The listing builds one solid part. Answer for the finished solid, in the listing's coordinates (mm). Coordinates: 2 decimals unless noted, no trailing zeros. Loops run counter-clockwise (first coordinate to the right, second up) from the corner with the lowest first, then second, coordinate; pieces in that order, holes last. Notation, with made-up numbers: (61, 11) - (74, 11) arc R6 cw to (74, 18) - close; hole circle Ø9 at (78, -38). An arc over 180 degrees is marked (long way). Use one line per item in the form item = value. Start each with the question number.
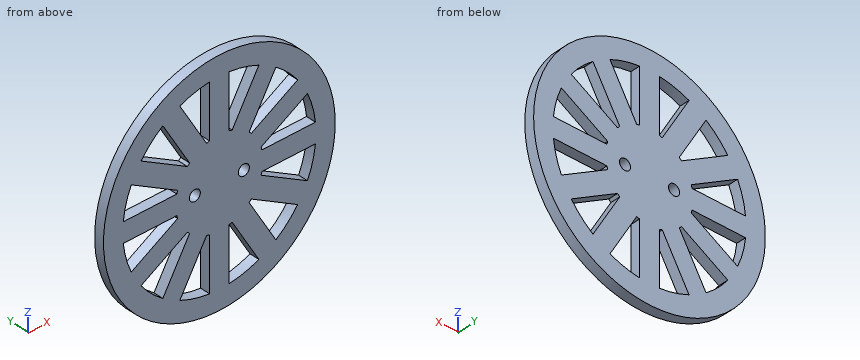
```python
from build123d import *

# Parameters (mm, degrees)
SKETCH1_R           = 30
SKETCH1_R_2         = 1.4224
BOSS_EXTRUDE1_DEPTH = 2.54


with BuildPart() as part:
    # Sketch1 → Boss-Extrude1 (new body)
    with BuildSketch(Plane(origin=(0, 0, 0), x_dir=(1, 0, 0), z_dir=(0, 1, 0))):
        Circle(SKETCH1_R)
        with BuildLine():
            ThreePointArc((3.308860999, 10.811115366), (2.926244071, 10.920891548), (2.54, 11.01713105))
            Line((2.54, 11.01713105), (2.54, 24.870633323))
            ThreePointArc((2.54, 24.870633323), (6.470476137, 24.148145694), (10.235612136, 22.808600266))
            Line((10.235612136, 22.808600266), (3.308860999, 10.811115366))
        make_face(mode=Mode.SUBTRACT)
        with BuildLine():
            ThreePointArc((8.271115366, 7.708270051), (7.994647477, 7.994647477), (7.708270051, 8.271115366))
            Line((7.708270051, 8.271115366), (14.635021187, 20.268600266))
            ThreePointArc((14.635021187, 20.268600266), (17.677669557, 17.677669557), (20.268600266, 14.635021187))
            Line((20.268600266, 14.635021187), (8.271115366, 7.708270051))
        make_face(mode=Mode.SUBTRACT)
        with BuildLine():
            ThreePointArc((11.01713105, 2.54), (10.920891548, 2.926244071), (10.811115366, 3.308860999))
            Line((10.811115366, 3.308860999), (22.808600266, 10.235612136))
            ThreePointArc((22.808600266, 10.235612136), (24.148145694, 6.470476137), (24.870633323, 2.54))
            Line((24.870633323, 2.54), (11.01713105, 2.54))
        make_face(mode=Mode.SUBTRACT)
        with BuildLine():
            ThreePointArc((10.811115366, -3.308860999), (10.920891548, -2.926244071), (11.01713105, -2.54))
            Line((11.01713105, -2.54), (24.870633323, -2.54))
            ThreePointArc((24.870633323, -2.54), (24.148145694, -6.470476137), (22.808600266, -10.235612136))
            Line((22.808600266, -10.235612136), (10.811115366, -3.308860999))
        make_face(mode=Mode.SUBTRACT)
        with BuildLine():
            ThreePointArc((7.708270051, -8.271115366), (7.994647477, -7.994647477), (8.271115366, -7.708270051))
            Line((8.271115366, -7.708270051), (20.268600266, -14.635021187))
            ThreePointArc((20.268600266, -14.635021187), (17.677669557, -17.677669557), (14.635021187, -20.268600266))
            Line((14.635021187, -20.268600266), (7.708270051, -8.271115366))
        make_face(mode=Mode.SUBTRACT)
        with BuildLine():
            ThreePointArc((2.54, -11.01713105), (2.926244071, -10.920891548), (3.308860999, -10.811115366))
            Line((3.308860999, -10.811115366), (10.235612136, -22.808600266))
            ThreePointArc((10.235612136, -22.808600266), (6.470476137, -24.148145694), (2.54, -24.870633323))
            Line((2.54, -24.870633323), (2.54, -11.01713105))
        make_face(mode=Mode.SUBTRACT)
        with BuildLine():
            ThreePointArc((-3.308860999, -10.811115366), (-2.926244071, -10.920891548), (-2.54, -11.01713105))
            Line((-2.54, -11.01713105), (-2.54, -24.870633323))
            ThreePointArc((-2.54, -24.870633323), (-6.470476137, -24.148145694), (-10.235612136, -22.808600266))
            Line((-10.235612136, -22.808600266), (-3.308860999, -10.811115366))
        make_face(mode=Mode.SUBTRACT)
        with BuildLine():
            ThreePointArc((-8.271115366, -7.708270051), (-7.994647477, -7.994647477), (-7.708270051, -8.271115366))
            Line((-7.708270051, -8.271115366), (-14.635021187, -20.268600266))
            ThreePointArc((-14.635021187, -20.268600266), (-17.677669557, -17.677669557), (-20.268600266, -14.635021187))
            Line((-20.268600266, -14.635021187), (-8.271115366, -7.708270051))
        make_face(mode=Mode.SUBTRACT)
        with BuildLine():
            ThreePointArc((-11.01713105, -2.54), (-10.920891548, -2.926244071), (-10.811115366, -3.308860999))
            Line((-10.811115366, -3.308860999), (-22.808600266, -10.235612136))
            ThreePointArc((-22.808600266, -10.235612136), (-24.148145694, -6.470476137), (-24.870633323, -2.54))
            Line((-24.870633323, -2.54), (-11.01713105, -2.54))
        make_face(mode=Mode.SUBTRACT)
        with BuildLine():
            ThreePointArc((-10.811115366, 3.308860999), (-10.920891548, 2.926244071), (-11.01713105, 2.54))
            Line((-11.01713105, 2.54), (-24.870633323, 2.54))
            ThreePointArc((-24.870633323, 2.54), (-24.148145694, 6.470476137), (-22.808600266, 10.235612136))
            Line((-22.808600266, 10.235612136), (-10.811115366, 3.308860999))
        make_face(mode=Mode.SUBTRACT)
        with BuildLine():
            ThreePointArc((-7.708270051, 8.271115366), (-7.994647477, 7.994647477), (-8.271115366, 7.708270051))
            Line((-8.271115366, 7.708270051), (-20.268600266, 14.635021187))
            ThreePointArc((-20.268600266, 14.635021187), (-17.677669557, 17.677669557), (-14.635021187, 20.268600266))
            Line((-14.635021187, 20.268600266), (-7.708270051, 8.271115366))
        make_face(mode=Mode.SUBTRACT)
        with BuildLine():
            ThreePointArc((-2.54, 11.01713105), (-2.926244071, 10.920891548), (-3.308860999, 10.811115366))
            Line((-3.308860999, 10.811115366), (-10.235612136, 22.808600266))
            ThreePointArc((-10.235612136, 22.808600266), (-6.470476137, 24.148145694), (-2.54, 24.870633323))
            Line((-2.54, 24.870633323), (-2.54, 11.01713105))
        make_face(mode=Mode.SUBTRACT)
        with Locations((-6.35, 0)):
            Circle(SKETCH1_R_2, mode=Mode.SUBTRACT)
        with Locations((6.35, 0)):
            Circle(SKETCH1_R_2, mode=Mode.SUBTRACT)
    extrude(amount=BOSS_EXTRUDE1_DEPTH)


solid = part.part
```
(1) A cutting plane is placed at D-D (y = 1.1). State how many separate pieces and enclosed holes the cut face has, then the cut area to 3 significant figures.
(2) A cutting plane is placed at C-C (x = 13.5). Determine the outline of the cut face in (y, z).
(3) A cutting plane is placed at B-B (x = -24). Determine the outline of the cut face in (y, z), then the cut area to 3 significant figures.
(4) A cutting plane is placed at A-A (z = 0). Determine the outline of the cut face in (x, y).
(5) Find the intervals of material crossed by probe 1 along X at (y, z) = (1.25, 0); probe 2 along X at (y, z) = (1.4, -8.5); probe 3 along Z at (x, y) = (-22, 0.85), in increasing order. Write a range as from..to.
(6) Each of these flat-tipped pins is pushed along its axis until it touches: pin 1 Ø1.3 at (x, y) = (-19.5, 1) entering from +Z; pin 2 Ø10 at (x, z) = (-8.5, 21) entering from -Y; pin 3 Ø1.5 at (y, z) = (2, -7) entering from -X; pin 4 Ø1 at (y, z) = (1, 6) entering from +X. Where does it stop, or does it pass through?
Evaluation:
q1.separate_pieces = 1
q1.enclosed_holes = 14
q1.area = 2,090 mm^2
q2.outline = (0, -26.79) - (2.54, -26.79) - (2.54, -18.3) - (0, -18.3) - close; (0, -10.73) - (2.54, -10.73) - (2.54, -4.86) - (0, -4.86) - close; (0, -2.54) - (2.54, -2.54) - (2.54, 2.54) - (0, 2.54) - close; (0, 4.86) - (2.54, 4.86) - (2.54, 10.73) - (0, 10.73) - close; (0, 18.3) - (2.54, 18.3) - (2.54, 26.79) - (0, 26.79) - close
q3.outline = (0, -18) - (2.54, -18) - (2.54, -7) - (0, -7) - close; (0, -2.54) - (2.54, -2.54) - (2.54, 2.54) - (0, 2.54) - close; (0, 7) - (2.54, 7) - (2.54, 18) - (0, 18) - close
q3.area = 68.8 mm^2
q4.outline = (-30, 0) - (-7.77, 0) - (-7.77, 2.54) - (-30, 2.54) - close; (-4.93, 0) - (4.93, 0) - (4.93, 2.54) - (-4.93, 2.54) - close; (7.77, 0) - (30, 0) - (30, 2.54) - (7.77, 2.54) - close
q5.probe_1 = -30..-7.77, -4.93..4.93, 7.77..30
q5.probe_2 = -28.77..-23.51, -19.8..-9.64, -7.84..7.84, 9.64..19.8, 23.51..28.77
q5.probe_3 = -20.4..-9.77, -2.54..2.54, 9.77..20.4
q6.pin_1 = 23.34
q6.pin_2 = 0
q6.pin_3 = -29.34
q6.pin_4 = 29.49
